```python
from build123d import *

# Parameters (mm, degrees)
SKETCH1_W           = 980
SKETCH1_H           = 420
BOSS_EXTRUDE1_DEPTH = 200
SKETCH2_W           = 700
SKETCH2_H           = 60
CUT_EXTRUDE1_DEPTH  = 420
SKETCH3_W           = 140
SKETCH3_H           = 420
BOSS_EXTRUDE2_DEPTH = 420
SKETCH4_R           = 100
CUT_EXTRUDE2_DEPTH  = 200
SKETCH5_R           = 60
CUT_EXTRUDE3_DEPTH  = 200
FILLET1_RADIUS      = 210
FILLET1_LENGTH      = 140
FILLET2_R           = 50
FILLET3_R           = 50


with BuildPart() as part:
    # Sketch1 → Boss-Extrude1 (new body)
    with BuildSketch(Plane(origin=(0, 0, 0), x_dir=(1, 0, 0), z_dir=(0, 1, 0))):
        with Locations((490, 210)):
            Rectangle(SKETCH1_W, SKETCH1_H)
    extrude(amount=BOSS_EXTRUDE1_DEPTH)

    # Sketch2 → Cut-Extrude1 (cut)
    with BuildSketch(Plane.XY):
        with Locations((490, 30)):
            Rectangle(SKETCH2_W, SKETCH2_H)
    extrude(amount=-CUT_EXTRUDE1_DEPTH, mode=Mode.SUBTRACT)

    # Sketch3 → Boss-Extrude2 (add)
    with BuildSketch(Plane.XY):
        with Locations((490, 410)):
            Rectangle(SKETCH3_W, SKETCH3_H)
    extrude(amount=-BOSS_EXTRUDE2_DEPTH)

    # Sketch4 → Cut-Extrude2 (cut)
    with BuildSketch(Plane(origin=(560, 0, 0), x_dir=(0, 0, -1), z_dir=(1, 0, 0))):
        with Locations((210, 410)):
            Circle(SKETCH4_R)
    extrude(amount=-CUT_EXTRUDE2_DEPTH, mode=Mode.SUBTRACT)

    # Sketch5 → Cut-Extrude3 (cut)
    with BuildSketch(Plane(origin=(0, 200, 0), x_dir=(1, 0, 0), z_dir=(0, 1, 0))):
        with Locations(Location((770, 210, 0), (0, 0, 270))):
            Circle(SKETCH5_R)
        with Locations(Location((210, 210, 0), (0, 0, 90))):
            Circle(SKETCH5_R)
    extrude(amount=-CUT_EXTRUDE3_DEPTH, mode=Mode.SUBTRACT)

    # Fillet1: full round fillet: the end face becomes a half cylinder, R = half its width
    fillet1_face = Plane((490, 620, -210), x_dir=(1, 0, 0), z_dir=(0, 1, 0))  # on the end face: x along it, z out of the body
    fillet1_slab = fillet1_face.offset(-FILLET1_RADIUS / 2) * Box(FILLET1_LENGTH, 2 * FILLET1_RADIUS, FILLET1_RADIUS, mode=Mode.PRIVATE)  # the body's end, R deep
    fillet1_round = Plane((490, 410, -210), x_dir=(0, 1, 0), z_dir=(1, 0, 0)) * Cylinder(FILLET1_RADIUS, FILLET1_LENGTH, mode=Mode.PRIVATE)  # its axis R under the face
    add(fillet1_slab - fillet1_round, mode=Mode.SUBTRACT)

    # Fillet2
    fillet2_edges = [part.edges().sort_by_distance(p)[0] for p in [
        (980, 200, -210),
    ]]
    fillet(fillet2_edges, radius=FILLET2_R)

    # Fillet3
    fillet3_edges = [part.edges().sort_by_distance(p)[0] for p in [
        (0, 200, -210),
    ]]
    fillet(fillet3_edges, radius=FILLET3_R)


solid = part.part
```
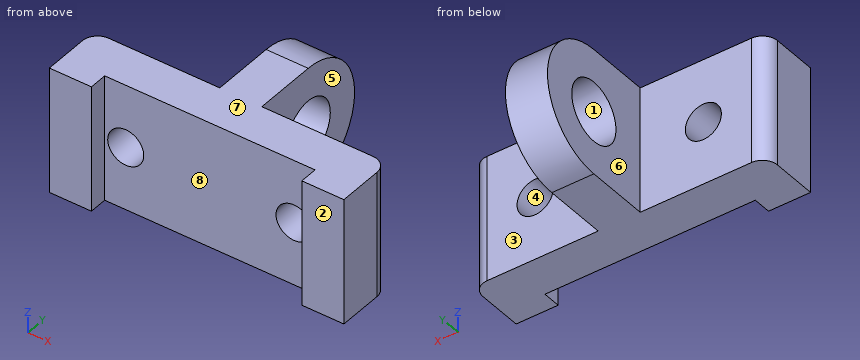
Input: part model. Units: mm. Frame: model coordinates. Face numbers are marked on the shaded views. A direction names the side the tool comes from. Give positions to 0.01 mm unless a question says otherwise; leave off trailing zeros. Loops run counter-clockwise (first coordinate to the right, second up) from the corner with the lowest first, then second, coordinate; pieces in that order, holes last.
1) Section query D-D on y = 123. Return the cut outline in (x, z).
A:
outline: (0, -420) - (980, -420) - (980, 0) - (0, 0) - close; hole circle Ø120 at (210, -210); hole circle Ø120 at (770, -210)
2) Contact query for flat-ended pins moving along their axis: pin 1 (1 mm diameter, centred on x = 307, z = -366.5, fed in from +Y); pin 2 (6 mm diameter, centred on x = 450, z = -68, fed in from +Y); pin 3 (6 mm diameter, centred on x = 522.5, z = -66, fed in from -Y). Output: stop coordinate, or through.
A:
pin 1: stops at y = 200
pin 2: stops at y = 567.41
pin 3: stops at y = 60
3) Line query: L1, parallel to Y at x = 412, z = -63; L2, parallel to X at y = 261, z = -371; L3, parallel to Z at x = 210, y = 170. Output: solid intervals per line, ascending.
A:
L1: y = 60 to 200
L2: x = 420 to 560
L3: z = -420 to -270, -150 to 0
4) Mould query, pull axis Y, two halves, no side actions, for the marked faces 1, 2, 3 and 4. Classes: released by +Y, released by -Y, zero draft, split by the parting line, or undercut.
A:
face 1: undercut
face 2: released by -Y
face 3: released by +Y
face 4: zero draft
5) Section query A-A on z = -210. Return the cut outline in (x, y), and give its area (3 significant figures).
A:
outline: (0, 0) - (140, 0) - (140, 60) - (150, 60) - (150, 200) - (50, 200) arc R50 ccw to (0, 150) - close; (270, 60) - (710, 60) - (710, 200) - (560, 200) - (560, 310) - (420, 310) - (420, 200) - (270, 200) - close; (420, 510) - (560, 510) - (560, 620) - (420, 620) - close; (830, 60) - (840, 60) - (840, 0) - (980, 0) - (980, 150) arc R50 ccw to (930, 200) - (830, 200) - close
area: 150,000 mm2
6) Section query C-C on x = 210. Return the cut outline in (y, z), and give its area (3 significant figures).
A:
outline: (60, -420) - (200, -420) - (200, -270) - (60, -270) - close; (60, -150) - (200, -150) - (200, 0) - (60, 0) - close
area: 42,000 mm2
7) Section query B-B on y = 49. Return the cut outline in (x, z).
A:
outline: (0, -420) - (140, -420) - (140, 0) - (0, 0) - close; (840, -420) - (980, -420) - (980, 0) - (840, 0) - close
8) Reachability of the marked faces 5, 6, 7 and 8 from +Z, -Z, +X, -X, +Y, -Y: full face, straight path, thin tool, end or side. Return the list, or none.
A:
face 5: +Z, -Z, +X, +Y
face 6: +Z, -Z, -X, +Y
face 7: +Z, +X, -X, +Y, -Y
face 8: +Z, -Z, -Y
